Drawing for the job (mm, zero at the part's lowest x, y, z). A direction names the side the tool comes from. Round coordinates to 2 decimals unless told otherwise and drop trailing zeros. Write each loop counter-clockwise with the first axis right and the second up, starting at its lowest first coordinate (ties: lowest second). Pieces come first, ordered by that corner, then holes.
Item 1: Band-saw the part on C-C, the plane x = 91.5. Write the cut outline in (y, z).
Item 2: Band-saw the part on B-B, the plane z = 9. Write the cut outline in (x, y).
Item 3: Band-saw the part on D-D, the plane x = 62. Write the cut outline in (y, z), then the cut area to 3 significant figures.
Item 4: Drop flat-ended pins along their axis: pin 1 Ø6 at (x, z) = (27, 33) entering from +Y; pin 2 Ø16 at (x, y) = (10, 40) entering from +Z; pin 3 Ø13 at (x, y) = (10, 10) entering from +Z. Give the stop position or say it passes through.
Item 5: 3-axis set-ups, long thin cutter, end or side, ignore diameter. For the marked faces 1, 2 and 3: which of +Z, -Z, +X, -X, +Y, -Y reach the whole face in a straight line?
Item 6: Wall check: probe 1 along Y at (x, z) = (90, 3.5); probe 2 along X at (y, z) = (10.5, 2.5); probe 3 along Y at (x, z) = (14, 24). Give the ranges that are in metal, low to high.
Item 7: Band-saw the part on A-A, the plane y = 10. Write the cut outline in (x, z).
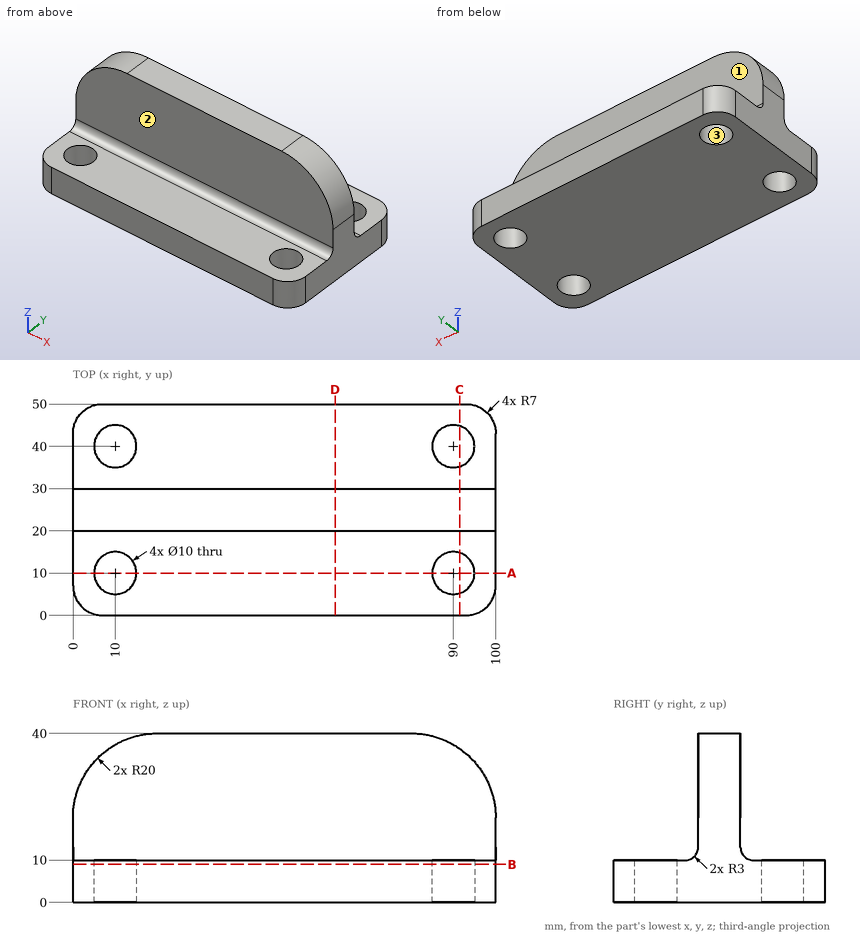
Results:
1. outline: (0, 0) - (5.23, 0) - (5.23, 10) - (0, 10) - close; (14.77, 0) - (35.23, 0) - (35.23, 10) - (33, 10) arc R3 cw to (30, 13) - (30, 36.36) - (20, 36.36) - (20, 13) arc R3 cw to (17, 10) - (14.77, 10) - close; (44.77, 0) - (50, 0) - (50, 10) - (44.77, 10) - close
2. outline: (0, 7) arc R7 ccw to (7, 0) - (93, 0) arc R7 ccw to (100, 7) - (100, 43) arc R7 ccw to (93, 50) - (7, 50) arc R7 ccw to (0, 43) - close; hole circle Ø10 at (10, 10); hole circle Ø10 at (10, 40); hole circle Ø10 at (90, 10); hole circle Ø10 at (90, 40)
3. outline: (0, 0) - (50, 0) - (50, 10) - (33, 10) arc R3 cw to (30, 13) - (30, 40) - (20, 40) - (20, 13) arc R3 cw to (17, 10) - (0, 10) - close
3. area: 804 mm2
4. pin 1: stops at y = 30
4. pin 2: stops at z = 10.17
4. pin 3: stops at z = 10
5. face 1: +Z, +X, -X, +Y
5. face 2: +Z, +X, -X, -Y
5. face 3: +Z, -Z
6. probe 1: y = 0 to 5, 15 to 35, 45 to 50
6. probe 2: x = 0 to 5.03, 14.97 to 85.03, 94.97 to 100
6. probe 3: y = 20 to 30
7. outline: (0, 0) - (5, 0) - (5, 10) - (0, 10) - close; (15, 0) - (85, 0) - (85, 10) - (15, 10) - close; (95, 0) - (100, 0) - (100, 10) - (95, 10) - close
